from build123d import *

# Parameters (mm, degrees)
FILLET1_R           = 1.5
SKETCH2_R           = 1
CUT_EXTRUDE1_DEPTH  = 5
BOSS_EXTRUDE1_DEPTH = 1


with BuildPart() as part:
    # Sketch1 → Revolve1 (revolve)
    with BuildSketch(Plane(origin=(0, 0, 0), x_dir=(1, 0, 0), z_dir=(0, 1, 0))):
        with BuildLine():
            Line((0.095371477, 16.5), (-1.404628523, 16.5))
            Line((-1.404628523, 16.5), (-1.404628523, 15))
            Line((-1.404628523, 15), (-10.044628523, 15))
            Line((-10.044628523, 15), (-10.044628523, 13))
            Line((-10.044628523, 13), (-7.631517886, 13))
            Line((-7.631517886, 13), (-7.631517886, 3.5))
            Line((-7.631517886, 3.5), (-10.044628523, 3.5))
            Line((-10.044628523, 3.5), (-10.044628523, 1.5))
            Line((-10.044628523, 1.5), (-7.631517886, 1.5))
            Line((-7.631517886, 1.5), (-2.613091993, 1.5))
            Line((-2.613091993, 1.5), (-2.613091993, 8.5))
            Line((-2.613091993, 8.5), (-4.113091993, 10))
            Line((-4.113091993, 10), (-4.113091993, 10.5))
            Line((-4.113091993, 10.5), (-3.613091993, 10.5))
            Line((-3.613091993, 10.5), (-3.613091993, 12.570770776))
            Line((-3.613091993, 12.570770776), (-1.543093741, 12.863761539))
            ThreePointArc((-1.543093741, 12.863761539), (0.164689844, 14.281505523), (0.095371477, 16.5))
        make_face()
    revolve(axis=Axis((-25, 0, 0), (1, 0, 0)))

    # Fillet1
    fillet1_edges = [part.edges().sort_by_distance(p)[0] for p in [
        (-2.613091993, 0, 8.5),
    ]]
    fillet(fillet1_edges, radius=FILLET1_R)

    # Sketch2 → Cut-Extrude1 (cut, symmetric)
    with BuildSketch(Plane(origin=(-2.613091993, 0, 0), x_dir=(0, 0, -1), z_dir=(1, 0, 0))):
        with Locations((0, 5)):
            Circle(SKETCH2_R)
        with Locations((5, 0)):
            Circle(SKETCH2_R)
        with Locations((0, -5)):
            Circle(SKETCH2_R)
        with Locations((-5, 0)):
            Circle(SKETCH2_R)
    extrude(amount=CUT_EXTRUDE1_DEPTH, both=True, mode=Mode.SUBTRACT)

    # Sketch3 → Boss-Extrude1 (add)
    with BuildSketch(Plane(origin=(-3.613091993, 0, 0), x_dir=(0, 0, -1), z_dir=(1, 0, 0))):
        Polygon((8.43091754, 7.253822764), (9.041610985, 7.95188113), (8.742421428, 8.82978635), (7.832538427, 9.009633204), (7.221844982, 8.311574837), (7.521034539, 7.433669617), align=None)
        Polygon((0.832331699, 11.09078623), (0.77055537, 12.016213511), (-0.061776329, 12.425427281), (-0.832331699, 11.90921377), (-0.77055537, 10.983786489), (0.061776329, 10.574572719), align=None)
        Polygon((11.09078623, -0.832331699), (12.016213511, -0.77055537), (12.425427281, 0.061776329), (11.90921377, 0.832331699), (10.983786489, 0.77055537), (10.574572719, -0.061776329), align=None)
        Polygon((7.253822764, -8.43091754), (7.95188113, -9.041610985), (8.82978635, -8.742421428), (9.009633204, -7.832538427), (8.311574837, -7.221844982), (7.433669617, -7.521034539), align=None)
        Polygon((-0.832331699, -11.09078623), (-0.77055537, -12.016213511), (0.061776329, -12.425427281), (0.832331699, -11.90921377), (0.77055537, -10.983786489), (-0.061776329, -10.574572719), align=None)
        Polygon((-8.43091754, -7.253822764), (-9.041610985, -7.95188113), (-8.742421428, -8.82978635), (-7.832538427, -9.009633204), (-7.221844982, -8.311574837), (-7.521034539, -7.433669617), align=None)
        Polygon((-11.09078623, 0.832331699), (-12.016213511, 0.77055537), (-12.425427281, -0.061776329), (-11.90921377, -0.832331699), (-10.983786489, -0.77055537), (-10.574572719, 0.061776329), align=None)
        Polygon((-7.253822764, 8.43091754), (-7.95188113, 9.041610985), (-8.82978635, 8.742421428), (-9.009633204, 7.832538427), (-8.311574837, 7.221844982), (-7.433669617, 7.521034539), align=None)
    extrude(amount=BOSS_EXTRUDE1_DEPTH)


solid = part.part
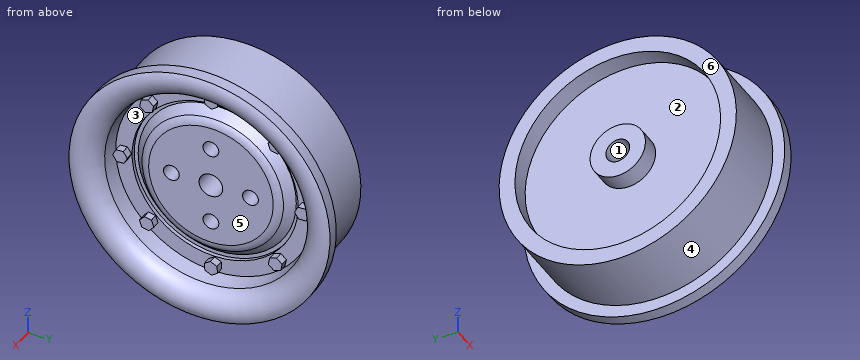
Input: part model. Units: mm. Frame: model coordinates. Face numbers are marked on the shaded views. A direction names the side the tool comes from. Coordinates: 2 decimals unless noted, no trailing zeros. Order: outer loops, then holes, each group sorted by start corner. A loop starts at its lowest first (then second) coordinate and runs counter-clockwise, first axis right, second up.
1. Ray query, line 1 along Y through (x, z) = (-5.5, 0); line 2 along Y through (x, z) = (-8.6, 0); line 3 along Y through (x, z) = (-3.8, 0). Return the intervals inside material, ascending.
Checked values:
line 1: y = -15 to -6, -4 to -1.5, 1.5 to 4, 6 to 15
line 2: y = -15 to -13, -3.5 to -1.5, 1.5 to 3.5, 13 to 15
line 3: y = -15 to -10.5, -9.69 to -6, -4 to -1.5, 1.5 to 4, 6 to 9.69, 10.5 to 15
2. Access query for the marked faces 1, 2 and 3. Directions: +Z, -Z, +X, -X, +Y, -Y. A direction counts if a zero-diameter tool reaches every point of the face in a straight line with its end or side. Return the directions, or none.
Checked values:
face 1: +X, -X
face 2: -X
face 3: +X
3. Draft query along Z for the marked faces 4, 5 and 6. Return one class per face: +Z half, -Z half, draft (parallel to the pull), parting line (faces both ways), or undercut.
Checked values:
face 4: parting line
face 5: undercut
face 6: draft
4. Cut plane A-A, the plane x = -5.75. Return loops of the section in (y, z), plus the area to 3 significant figures.
Checked values:
outline: circle Ø30 at (0, 0); hole circle Ø2 at (-5, 0); hole circle Ø3 at (0, 0); hole circle Ø2 at (0, -5); hole circle Ø2 at (0, 5); hole circle Ø2 at (5, 0)
area: 687 mm2
5. Contact query for flat-ended pins moving along their axis: P1, Ø1, axis at y = -5.5, z = 0.5, coming from the +X side; P2, Ø1, axis at x = -2.5, z = -7.5, coming from the -Y side; P3, Ø1, axis at x = -8, z = 2.5, coming from the -Y side; P4, Ø4, axis at y = 0, z = 0, coming from the -X side. Output: stop coordinate, or through.
Checked values:
P1: stops at x = -2.61
P2: stops at y = -13.27
P3: stops at y = -14.87
P4: stops at x = -10.04
